Geometry: see drawing. Coordinates: mm, zero at the bounding-box minimum. Round coordinates to 2 decimals unless told otherwise and drop trailing zeros. Loops run counter-clockwise (first coordinate to the right, second up) from the corner with the lowest first, then second, coordinate; pieces in that order, holes last. Notation, with made-up numbers: (54, -17.75) -> (66, -17.75) arc R22 cw to (66, 1.25) -> close; hole circle Ø5 at (52.25, 40.5). An arc over 180 degrees is marked (long way). Write item = value, one per line.
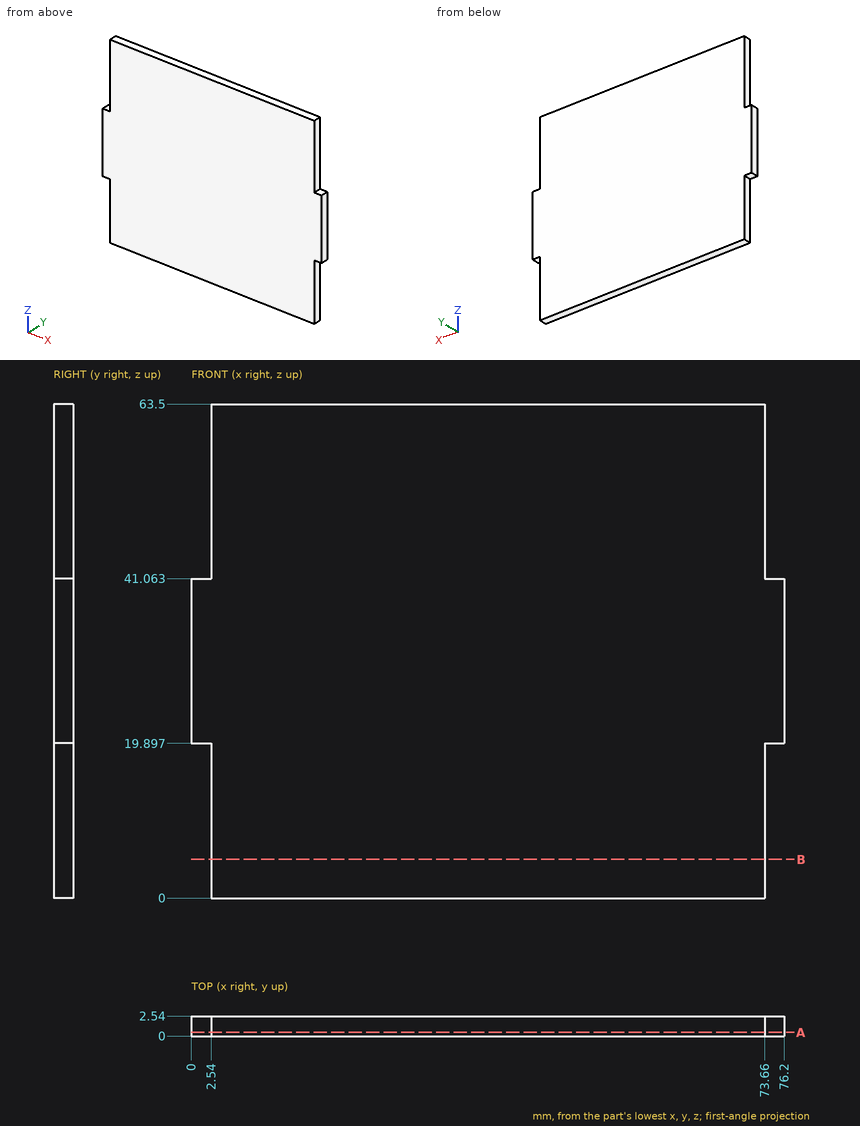
1. Contact query for flat-ended pins moving along their axis: pin 1 Ø1.3 at (x, y) = (74.5, 1.5) entering from -Z; pin 2 Ø0.8 at (y, z) = (1.5, 6.5) entering from -X; pin 3 Ø0.8 at (y, z) = (2, 48.5) entering from +X. Output: stop coordinate, or through.
Evaluation:
pin_1 = 19.9
pin_2 = 2.54
pin_3 = 73.66
2. Section query A-A (y = 0.45). Return the cut outline in (x, z), then the cut area to 3 significant figures.
Evaluation:
outline = (0, 19.9) -> (2.54, 19.9) -> (2.54, 0) -> (73.66, 0) -> (73.66, 19.9) -> (76.2, 19.9) -> (76.2, 41.06) -> (73.66, 41.06) -> (73.66, 63.5) -> (2.54, 63.5) -> (2.54, 41.06) -> (0, 41.06) -> close
area = 4,620 mm²
3. Section query B-B (z = 5). Return the cut outline in (x, y), then the cut area to 3 significant figures.
Evaluation:
outline = (2.54, 0) -> (73.66, 0) -> (73.66, 2.54) -> (2.54, 2.54) -> close
area = 181 mm²
4. Line query: probe 1 along X at (y, z) = (2.35, 53.5). Output: solid intervals per line, ascending. Write a range as from..to.
Evaluation:
probe_1 = 2.54..73.66
